from build123d import *

# Parameters (mm, degrees)
SKETCH_2_R          = 16
CUT_EXTRUDE_1_DEPTH = 11
SKETCH_3_W          = 1.5
SKETCH_3_H          = 1.5


with BuildPart() as part:
    # 草图1 → 旋转1 (revolve)
    with BuildSketch(Plane(origin=(0, 0, 0), x_dir=(1, 0, 0), z_dir=(0, 1, 0))):
        with BuildLine():
            Line((13, 0), (28, 0))
            ThreePointArc((28, 0), (37.75, 9.75), (28, 19.5))
            Line((28, 19.5), (13, 19.5))
            Line((13, 19.5), (13, 0))
        make_face()
    revolve(axis=Axis((0, 0, 0), (0, 0, -1)))

    # 草图2 → 切除-拉伸1 (cut)
    with BuildSketch(Plane(origin=(0, 0, -19.5), x_dir=(-1, 0, 0), z_dir=(0, 0, -1))):
        Circle(SKETCH_2_R)
    extrude(amount=-CUT_EXTRUDE_1_DEPTH, mode=Mode.SUBTRACT)

    # 草图3 → 切除-旋转1 (revolve, cut)
    with BuildSketch(Plane(origin=(0, 0, 0), x_dir=(1, 0, 0), z_dir=(0, 1, 0)), mode=Mode.PRIVATE) as cut_revolve_1_sk:
        with Locations((16.75, 16.55)):
            Rectangle(SKETCH_3_W, SKETCH_3_H)
    revolve(cut_revolve_1_sk.sketch.rotate(Axis((0, 0, 0), (0, 0, -1)), 180), axis=Axis((0, 0, 0), (0, 0, -1)), mode=Mode.SUBTRACT)


solid = part.part
The model under review builds one solid part; all positions refer to its coordinate system, in mm. A direction names the side the tool comes from. Coordinates: 2 decimals unless noted, no trailing zeros. Loops run counter-clockwise (first coordinate to the right, second up) from the corner with the lowest first, then second, coordinate; pieces in that order, holes last. Notation, with made-up numbers: (70, -13) -> (109, -13) arc R36 ccw to (109, 26) -> close; hole circle Ø6 at (7.25, 81). An arc over 180 degrees is marked (long way). Use a Markdown table: item, result. Add a question column.
1. Add section D-D on z = -13.75. Write out the cut boundary in (x, y), plus the area to 3 significant figures.
2. Add section A-A on x = 0. Write out the cut boundary in (y, z), plus the area to 3 significant figures.
3. Machinability: for faces 1 (the face through (3.794, -17.084, -16.56)), 2 (the face through (3.47, -15.62, -12.2)), 3 (the face through (12, 12, -19.5)), which of the approach directions +Z, -Z, +X, -X, +Y, -Y give a long, thin tool a straight path to every point of the face, cutting with its end or side? Answer none if there is none.
4. Draft analysis for pull direction Y (two halves, no side actions). For faces 4 (the face through (-6, 12, 0)), 5 (the face through (3.47, -15.62, -18.42)), 6 (the face through (7.7, -14.2, -15.8)), state which applies: pulls with the +Y half, pulls with the -Y half, needs draft (parallel to the pull), parting line crosses it, or undercut.
5. To check wall thickness, follow line 1 (Z direction, x = 23, y = -16.5); line 2 (Y direction, x = 0, z = -12); line 3 (X direction, y = -1.5, z = -18). State the ranges of each line that lie inside material, in increasing order.
6. Add section C-C on z = -9.75. Write out the cut boundary in (x, y).
7. Clearance check with flat-ended pins moving along their axes: pin 1 Ø5 at (x, z) = (-30, -2.5) entering from -Y; pin 2 Ø5 at (y, z) = (19.5, -16) entering from +X; pin 3 Ø4 at (x, z) = (-4, -7) entering from +Y. State where each tip first meets the part, or that it passes through.
Returned:
| question | item | result |
|---|---|---|
| 1 | outline | circle Ø73.78 at (0, 0); hole circle Ø32 at (0, 0) |
| 1 | area | 3,470 mm² |
| 2 | outline | (-28, -19.5) -> (-16, -19.5) -> (-16, -17.3) -> (-17.5, -17.3) -> (-17.5, -15.8) -> (-16, -15.8) -> (-16, -8.5) -> (-13, -8.5) -> (-13, 0) -> (-28, 0) arc R9.75 ccw to start; (13, -8.5) -> (16, -8.5) -> (16, -15.8) -> (17.5, -15.8) -> (17.5, -17.3) -> (16, -17.3) -> (16, -19.5) -> (28, -19.5) arc R9.75 ccw to (28, 0) -> (13, 0) -> close |
| 2 | area | 813 mm² |
| 3 | face 1 | none |
| 3 | face 2 | -Z |
| 3 | face 3 | -Z, +X, -X, +Y, -Y |
| 4 | face 4 | needs draft |
| 4 | face 5 | undercut |
| 4 | face 6 | undercut |
| 5 | line 1 | z = -19.5 to 0 |
| 5 | line 2 | y = -37.49 to -16, 16 to 37.49 |
| 5 | line 3 | x = -33.16 to -15.93, 15.93 to 33.16 |
| 6 | outline | circle Ø75.5 at (0, 0); hole circle Ø32 at (0, 0) |
| 7 | pin 1 | stops at y = -22.45 |
| 7 | pin 2 | stops at x = 32.09 |
| 7 | pin 3 | stops at y = 37.58 |
